Input: part model. Units: mm. Frame: model coordinates. Face numbers are marked on the shaded views. A direction names the side the tool comes from. Round coordinates to 2 decimals unless told otherwise and drop trailing zeros. Loops run counter-clockwise (first coordinate to the right, second up) from the corner with the lowest first, then second, coordinate; pieces in that order, holes last.
1) Section C-C, the plane y = 7. Return loops of the section in (x, z).
2) Access query for the marked faces 4, 5 and 6. Directions: +Z, -Z, +X, -X, +Y, -Y. A direction counts if a zero-diameter tool reaches every point of the face in a straight line with its end or side. Return the directions, or none.
3) Section D-D, the plane x = 26.5. Return loops of the section in (y, z).
4) First-contact query: pin 1 (1.5 mm diameter, centred on x = 25.5, y = 8, fed in from +Z); pin 2 (2.5 mm diameter, centred on x = 31.5, y = 15, fed in from +Z); pin 3 (8 mm diameter, centred on y = 14.5, z = -7, fed in from -X) (3 decimals); pin 4 (7 mm diameter, centred on x = 27, z = -38, fed in from +Y). Flat tips, straight axial feed; report the tip coordinate or a pass-through.
5) Section B-B, the plane z = -20. Return loops of the section in (x, y), and give its area (3 significant figures).
6) Section A-A, the plane x = 55.4. Return loops of the section in (y, z).
7) Ray query, line 1 along X through (y, z) = (4.75, -20); line 2 along X through (y, z) = (12, -20); line 3 along Z through (x, y) = (4.6, 8.25). Return the intervals inside material, ascending.
8) Draft query along X for the marked faces 1, 2 and 3. Return one class per face: pulls with the +X half, pulls with the -X half, needs draft (parallel to the pull), parting line crosses it, or undercut.
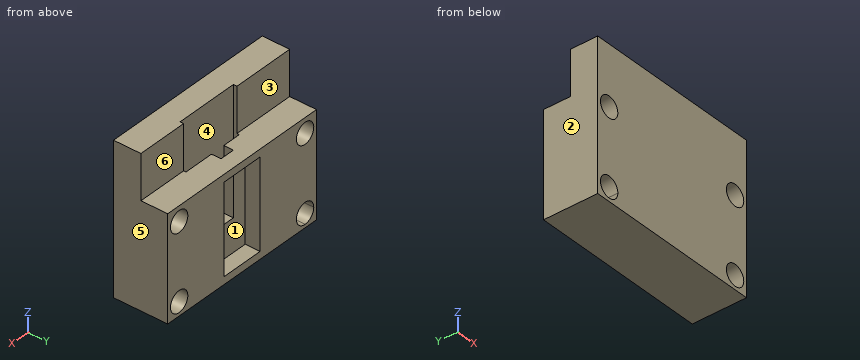
from build123d import *

# Parameters (mm, degrees)
SKETCH2_W               = 60
SKETCH2_H               = 50
BOSS_EXTRUDE1_DEPTH     = 10
SKETCH3_W               = 21.5
SKETCH3_H               = 36.5
CUT_EXTRUDE2_DEPTH      = 2
BOSS_EXTRUDE2_DEPTH     = 3.2
SKETCH5_W               = 60
SKETCH5_H               = 50
SKETCH5_W_2             = 14.5
SKETCH5_H_2             = 30
BOSS_EXTRUDE3_DEPTH     = 5
SKETCH1_R               = 3.5
CUT_EXTRUDE1_DEPTH      = 80.210100366
CUT_EXTRUDE1_DEPTH_BACK = 80.210100366
SKETCH7_W               = 60
SKETCH7_H               = 15
CUT_EXTRUDE3_DEPTH      = 9


with BuildPart() as part:
    # Sketch2 → Boss-Extrude1 (new body)
    with BuildSketch(Plane(origin=(0, 0, 0), x_dir=(1, 0, 0), z_dir=(0, 1, 0))):
        with Locations((30, 25)):
            Rectangle(SKETCH2_W, SKETCH2_H)
    extrude(amount=BOSS_EXTRUDE1_DEPTH)

    # Sketch3 → Cut-Extrude2 (cut)
    with BuildSketch(Plane(origin=(0, 10, 0), x_dir=(1, 0, 0), z_dir=(0, 1, 0))):
        with Locations((32, 18.25)):
            Rectangle(SKETCH3_W, SKETCH3_H)
    extrude(amount=-CUT_EXTRUDE2_DEPTH, mode=Mode.SUBTRACT)

    # Sketch4 → Boss-Extrude2 (add)
    with BuildSketch(Plane(origin=(0, 10, 0), x_dir=(1, 0, 0), z_dir=(0, 1, 0))):
        Polygon((27.5, 0), (27.5, 36.5), (32.5, 36.5), (32.5, 0), (60, 0), (60, 50), (0, 50), (0, 0), align=None)
    extrude(amount=BOSS_EXTRUDE2_DEPTH)

    # Sketch5 → Boss-Extrude3 (add)
    with BuildSketch(Plane(origin=(0, 13.2, 0), x_dir=(1, 0, 0), z_dir=(0, 1, 0))):
        with Locations((30, 25)):
            Rectangle(SKETCH5_W, SKETCH5_H)
        with Locations((30, 32.5)):
            Rectangle(SKETCH5_W_2, SKETCH5_H_2, mode=Mode.SUBTRACT)
    extrude(amount=BOSS_EXTRUDE3_DEPTH)

    # Sketch1 → Cut-Extrude1 (cut, two sides)
    with BuildSketch(Plane(origin=(0, 13.2, 0), x_dir=(1, 0, 0), z_dir=(0, 1, 0))) as cut_extrude1_sk:
        with BuildLine():
            Line((4.6, 48.9), (4.6, 45.4))
            Line((4.6, 45.4), (1.1, 45.4))
            ThreePointArc((1.1, 45.4), (4.6, 41.9), (8.1, 45.4))
            ThreePointArc((8.1, 45.4), (7.074873734, 47.874873734), (4.6, 48.9))
        make_face()
        with BuildLine():
            Line((1.1, 45.4), (4.6, 45.4))
            Line((4.6, 45.4), (4.6, 48.9))
            ThreePointArc((4.6, 48.9), (2.125126266, 47.874873734), (1.1, 45.4))
        make_face()
        with Locations(Location((55.4, 45.4, 0), (0, 0, 270))):
            Circle(SKETCH1_R)
        with Locations(Location((4.6, 20, 0), (0, 0, 270))):
            Circle(SKETCH1_R)
        with Locations(Location((55.4, 20, 0), (0, 0, 270))):
            Circle(SKETCH1_R)
    extrude(amount=CUT_EXTRUDE1_DEPTH, mode=Mode.SUBTRACT)
    extrude(cut_extrude1_sk.sketch, amount=-CUT_EXTRUDE1_DEPTH_BACK, mode=Mode.SUBTRACT)

    # Sketch7 → Cut-Extrude3 (cut)
    with BuildSketch(Plane(origin=(0, 18.2, 0), x_dir=(1, 0, 0), z_dir=(0, 1, 0))):
        with Locations((30, 7.5)):
            Rectangle(SKETCH7_W, SKETCH7_H)
    extrude(amount=-CUT_EXTRUDE3_DEPTH, mode=Mode.SUBTRACT)


solid = part.part
Final values:
1. outline: (0, -50) - (60, -50) - (60, 0) - (0, 0) - close; hole circle Ø7 at (4.6, -45.4); hole circle Ø7 at (4.6, -20); hole circle Ø7 at (55.4, -45.4); hole circle Ø7 at (55.4, -20)
2. face 4: +Z
2. face 5: +Z, -Z, +X, +Y, -Y
2. face 6: +Z, +X, -X, +Y
3. outline: (0, -50) - (18.2, -50) - (18.2, -47.5) - (13.2, -47.5) - (13.2, -17.5) - (18.2, -17.5) - (18.2, -15) - (10, -15) - (10, -36.5) - (8, -36.5) - (8, 0) - (0, 0) - close
4. pin 1: stops at z = 0
4. pin 2: stops at z = -15
4. pin 3: passes through
4. pin 4: stops at y = 13.2
5. outline: (0, 0) - (1.1, 0) - (1.1, 18.2) - (0, 18.2) - close; (8.1, 0) - (51.9, 0) - (51.9, 18.2) - (37.25, 18.2) - (37.25, 13.2) - (32.5, 13.2) - (32.5, 10) - (42.75, 10) - (42.75, 8) - (21.25, 8) - (21.25, 10) - (27.5, 10) - (27.5, 13.2) - (22.75, 13.2) - (22.75, 18.2) - (8.1, 18.2) - close; (58.9, 0) - (60, 0) - (60, 18.2) - (58.9, 18.2) - close
5. area: 706 mm2
6. outline: (0, -50) - (18.2, -50) - (18.2, -48.9) - (0, -48.9) - close; (0, -41.9) - (18.2, -41.9) - (18.2, -23.5) - (0, -23.5) - close; (0, -16.5) - (18.2, -16.5) - (18.2, -15) - (9.2, -15) - (9.2, 0) - (0, 0) - close
7. line 1: x = 0 to 1.1, 8.1 to 51.9, 58.9 to 60
7. line 2: x = 0 to 1.1, 8.1 to 27.5, 32.5 to 51.9, 58.9 to 60
7. line 3: z = -50 to -48.9, -41.9 to -23.5, -16.5 to 0
8. face 1: undercut
8. face 2: pulls with the -X half
8. face 3: needs draft
